Here's the drawing with two shaded views (mm, measured from the low corner). I have some questions. A direction names the side the tool comes from. Give positions to 0.01 mm unless a question says otherwise; leave off trailing zeros. Write each loop counter-clockwise with the first axis right and the second up, starting at its lowest first coordinate (ties: lowest second). Pieces come first, ordered by that corner, then holes. Notation, with made-up numbers: (71, 2) - (102, 2) arc R9 ccw to (102, 8) - close; hole circle Ø5 at (-8.5, -31). An arc over 180 degrees is marked (long way). Answer as CSV lines item,"result". Start each with the question number.
Q1. Imagine slicing it at B-B on z = 5. List the corners of the cut face in (x, y) for me.
Q2. Imagine slicing it at C-C on x = 5. List the corners of the cut face in (y, z) for me.
Q3. Imagine slicing it at D-D on z = 8. List the corners of the cut face in (x, y) for me.
Q4. Imagine slicing it at A-A on x = 41. List the corners of the cut face in (y, z) for me (1 decimal).
Q5. On a 3-axis mill with a long thin cutter (end or side, diameter ignored), from which of +Z, -Z, +X, -X, +Y, -Y can I reach the whole of each face in a straight line? I mean the marked faces 1, 2, 3 and 4. Say none if no direction works.
Q6. If I drill on line 1 along X through (y, z) = (1.05, 5); line 2 along Y through (x, z) = (41, 4.5); line 3 along Z through (x, y) = (5, 3), over which ranges is the centre line in solid material (lowest first)?
Q7. Will these pins go through, and if not, where does the flat tip stop? pin 1 Ø1.2 at (y, z) = (19.5, 5) entering from +X; pin 2 Ø18 at (x, y) = (31.5, 16) entering from -Z; pin 3 Ø4 at (x, y) = (16, 3) entering from +Z.
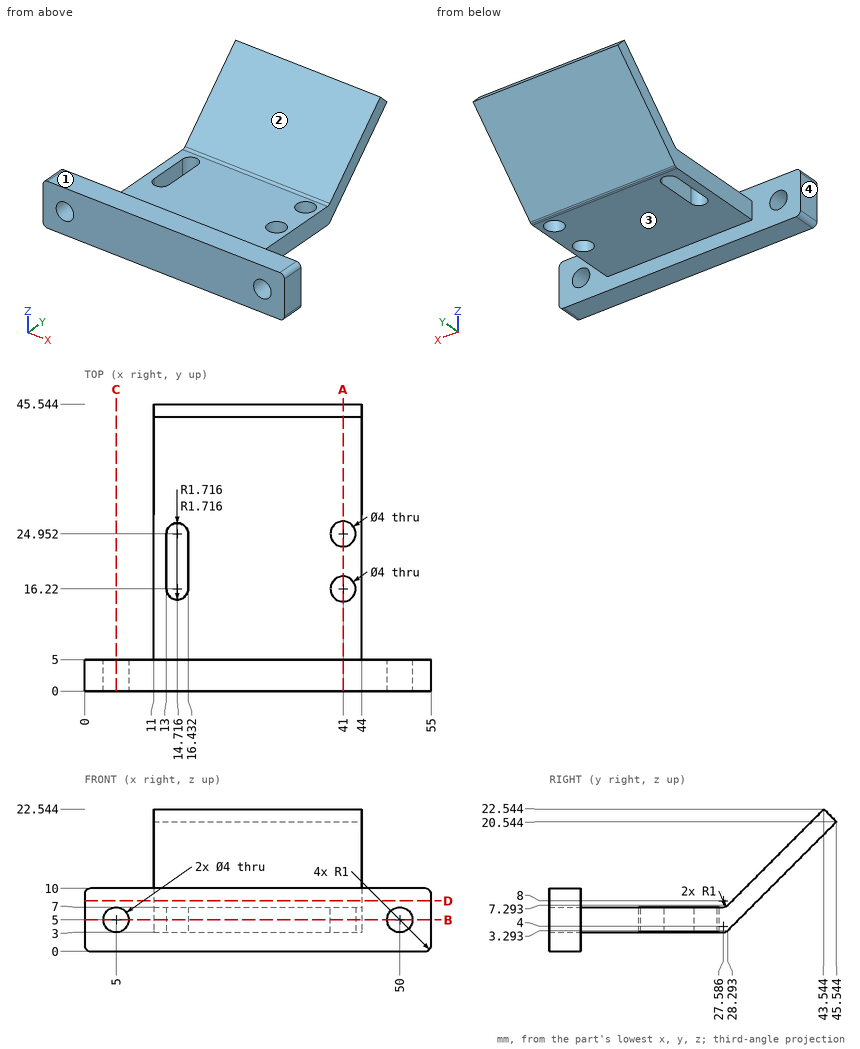
Conclusion:
1,outline,"(0, 0) - (3, 0) - (3, 5) - (0, 5) - close; (7, 0) - (48, 0) - (48, 5) - (44, 5) - (44, 30) - (11, 30) - (11, 5) - (7, 5) - close; (52, 0) - (55, 0) - (55, 5) - (52, 5) - close; hole (13, 16.22) arc R1.72 ccw to (16.43, 16.22) - (16.43, 24.95) arc R1.72 ccw to (13, 24.95) - close; hole circle Ø4 at (41, 16.22); hole circle Ø4 at (41, 24.95)"
2,outline,"(0, 0) - (5, 0) - (5, 3) - (0, 3) - close; (0, 7) - (5, 7) - (5, 10) - (0, 10) - close"
3,outline,"(0, 0) - (55, 0) - (55, 5) - (0, 5) - close; (11, 29) - (44, 29) - (44, 33) - (11, 33) - close"
4,outline,"(0, 0) - (5, 0) - (5, 3) - (14.2, 3) - (14.2, 7) - (5, 7) - (5, 10) - (0, 10) - close; (18.2, 3) - (23, 3) - (23, 7) - (18.2, 7) - close; (27, 3) - (27.6, 3) arc R1 ccw to (28.3, 3.3) - (45.5, 20.5) - (43.5, 22.5) - (28.3, 7.3) arc R1 cw to (27.6, 7) - (27, 7) - close"
5,face 1,"+Z, +X, -X, -Y"
5,face 2,"+Z, +X, -X"
5,face 3,"-Z, +X, -X, +Y"
5,face 4,"+Z, -Z, -X, +Y, -Y"
6,line 1,"0 to 3, 7 to 48, 52 to 55"
6,line 2,"0 to 14.22, 18.22 to 22.95, 26.95 to 29.5"
6,line 3,"0 to 3, 7 to 10"
7,pin 1,"x = 44"
7,pin 2,"z = 3"
7,pin 3,"z = 10"
